The figure shows three views and two pictorial views of one solid part (mm, origin at its lowest corner). Answer the questions. A direction names the side the tool comes from. Coordinates: 2 decimals unless noted, no trailing zeros. Order: outer loops, then holes, each group sorted by start corner. A loop starts at its lowest first (then second) coordinate and runs counter-clockwise, first axis right, second up.
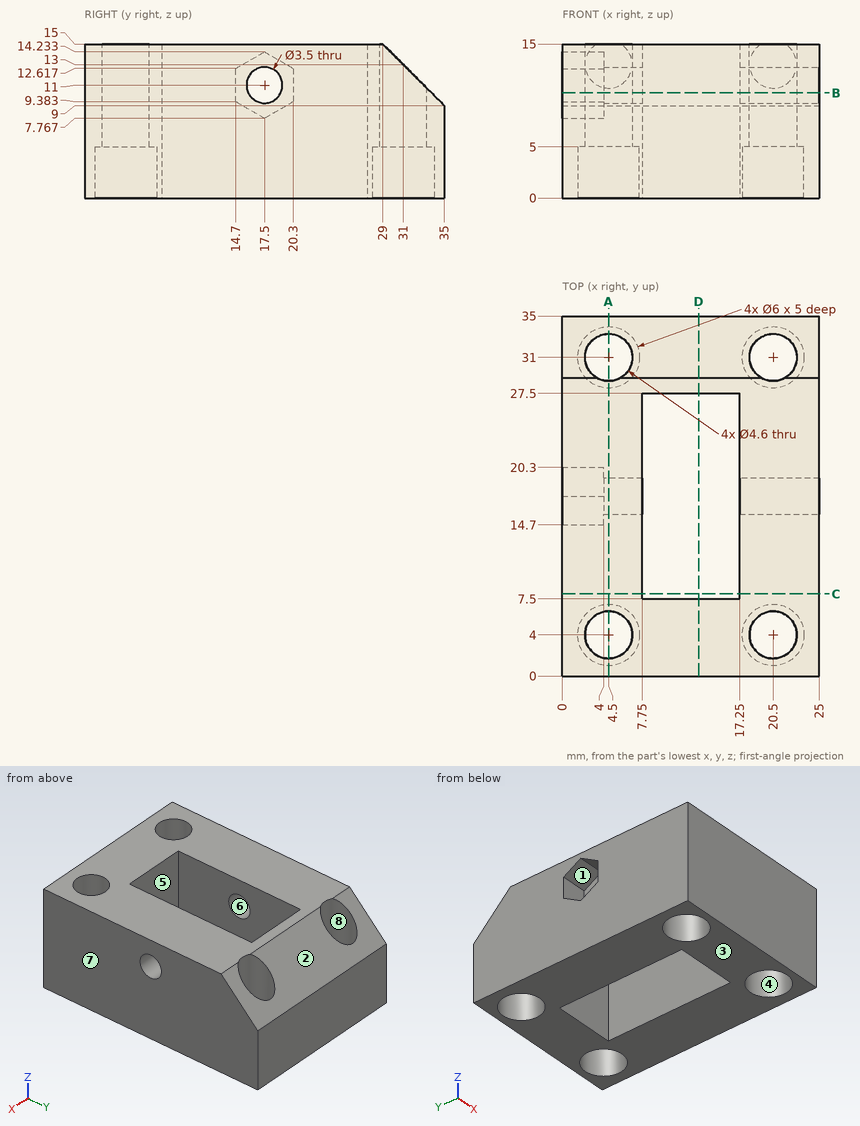
1) A cutting plane is placed at C-C, the plane y = 8. Write down the section's boundary in (x, z).
2) The mould has two halves that part along X. Classify the marked faces 6, 7 and 8: released by +X, released by -X, zero draft, split by the parting line, or undercut.
3) A cutting plane is placed at A-A, the plane x = 4.5. Write down the section's boundary in (y, z).
4) Each of these flat-tipped pins is pushed along its axis until it touches: P1, Ø1.8, axis at x = 3.5, y = 30.5, coming from the -Z side; P2, Ø5.5, axis at y = 17.5, z = 11, coming from the -X side. Where does it stop, or does it pass through?
5) Straight lines are drawn through the part: probe 1 along X at (y, z) = (4, 11); probe 2 along X at (y, z) = (31, 2.2); probe 3 along Y at (x, z) = (4.5, 3.75). For each, find the intervals that lie inside material, in ascending order.
6) For the marked faces 1, 2, 3, 4 and 5, determine the directions among +Z, -Z, +X, -X, +Y, -Y from which every point of the face is accessible in a straight line to the end or side of a thin tool.
7) A cutting plane is placed at D-D, the plane x = 13.25. Write down the section's boundary in (y, z), plus the area to 3 significant figures.
8) A cutting plane is placed at B-B, the plane z = 10.25. Write down the section's boundary in (x, y).
Working result:
1. outline: (0, 0) - (7.75, 0) - (7.75, 15) - (0, 15) - close; (17.25, 0) - (25, 0) - (25, 15) - (17.25, 15) - close
2. face 6: zero draft
2. face 7: released by +X
2. face 8: undercut
3. outline: (0, 0) - (1, 0) - (1, 5) - (1.7, 5) - (1.7, 15) - (0, 15) - close; (6.3, 5) - (7, 5) - (7, 0) - (28, 0) - (28, 5) - (28.7, 5) - (28.7, 15) - (6.3, 15) - close; (33.3, 5) - (34, 5) - (34, 0) - (35, 0) - (35, 9) - (33.3, 10.7) - close; hole circle Ø3.5 at (17.5, 11)
4. P1: passes through
4. P2: stops at x = 4
5. probe 1: x = 0 to 2.2, 6.8 to 18.2, 22.8 to 25
5. probe 2: x = 0 to 1.5, 7.5 to 17.5, 23.5 to 25
5. probe 3: y = 0 to 1, 7 to 28, 34 to 35
6. face 1: -X
6. face 2: +Z, +X, -X, +Y
6. face 3: -Z, +X, -X, +Y, -Y
6. face 4: -Z
6. face 5: +Z, -Z
7. outline: (0, 0) - (7.5, 0) - (7.5, 15) - (0, 15) - close; (27.5, 0) - (35, 0) - (35, 9) - (29, 15) - (27.5, 15) - close
7. area: 207 mm2
8. outline: (0, 0) - (25, 0) - (25, 15.92) - (17.25, 15.92) - (17.25, 7.5) - (7.75, 7.5) - (7.75, 15.92) - (4, 15.92) - (4, 14.7) - (0, 14.7) - close; (0, 20.3) - (4, 20.3) - (4, 19.08) - (7.75, 19.08) - (7.75, 27.5) - (17.25, 27.5) - (17.25, 19.08) - (25, 19.08) - (25, 33.75) - (0, 33.75) - close; hole circle Ø4.6 at (4.5, 4); hole circle Ø4.6 at (4.5, 31); hole circle Ø4.6 at (20.5, 4); hole circle Ø4.6 at (20.5, 31)
